For this review, use the dimensioned drawing (mm, ordinates from the lowest corner) and the shaded views. Give positions to 0.01 mm unless a question says otherwise; leave off trailing zeros. Write each loop counter-clockwise with the first axis right and the second up, starting at its lowest first coordinate (ties: lowest second). Pieces come first, ordered by that corner, then holes. Notation, with made-up numbers: (-6, 6) - (38, 6) arc R10 cw to (38, 18) - close; hole circle Ø5 at (25, 87). An arc over 180 degrees is marked (long way). One line per question, with ' | ' between items. Start each with the question number.
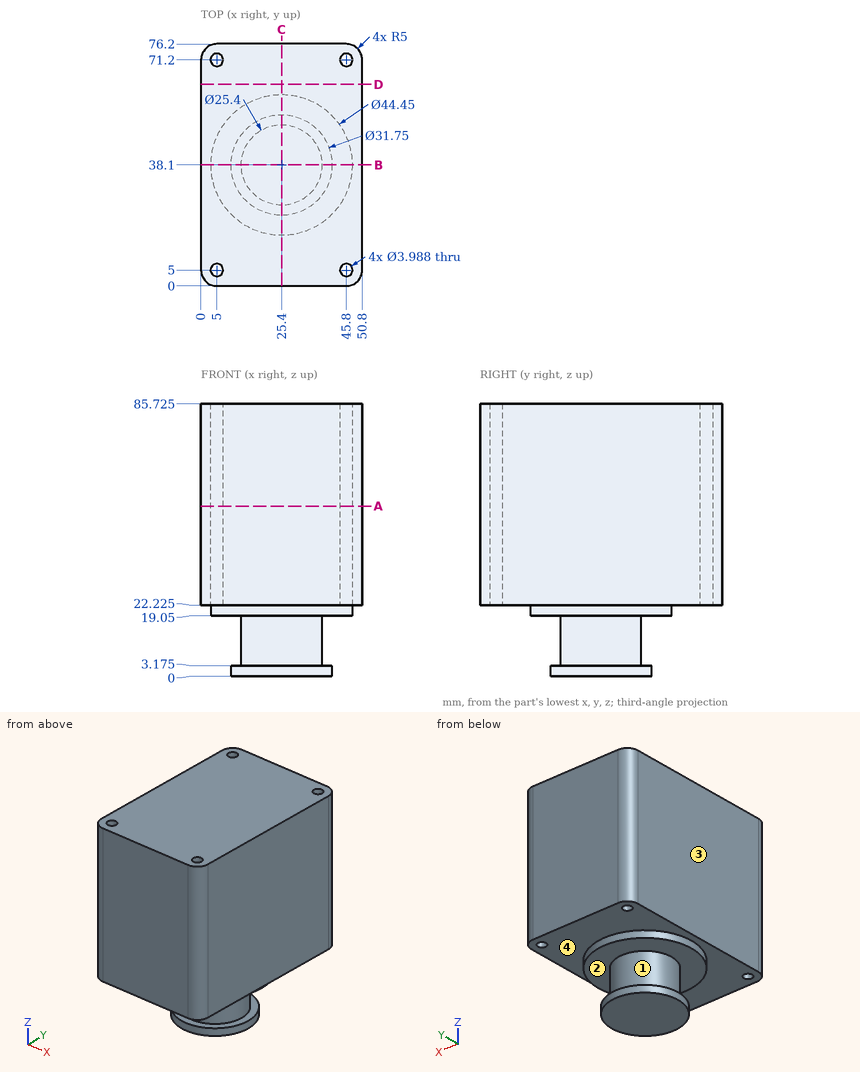
Item 1: Take a section at D-D (y = 63.5). Give the boundary of the cut face in (x, z) (3 decimals).
Item 2: The part is to be moulded in two halves that separate along Z. For the marked faces 1, 2, 3 and 4, say which applies: +Z half, -Z half, draft (parallel to the pull), parting line (faces both ways), or undercut.
Item 3: For probe 1 along Z at (x, y) = (36, 30) (3 decimals); probe 2 along Y at (x, z) = (6.5, 69); probe 3 along Z at (x, y) = (27.5, 64) (3 decimals), list the stretches that pass through material, from the lowest coordinate up.
Item 4: Take a section at B-B (y = 38.1). Give the boundary of the cut face in (x, z) (3 decimals), plus the area to 3 significant figures.
Item 5: Take a section at C-C (x = 25.4). Give the boundary of the cut face in (y, z) (3 decimals), plus the area to 3 significant figures.
Item 6: Clearance check with flat-ended pins moving along their axes: P1, Ø3.5, axis at x = 45.8, y = 71.2, coming from the +Z side; P2, Ø1, axis at x = 7, y = 43.5, coming from the -Z side. State where each tip first meets the part, or that it passes through.
Item 7: Take a section at A-A (z = 53.5). Give the boundary of the cut face in (x, y).
Check sheet entries:
1) outline: (0, 22.225) - (50.8, 22.225) - (50.8, 85.725) - (0, 85.725) - close
2) face 1: undercut | face 2: undercut | face 3: draft | face 4: -Z half
3) probe 1: z = 0 to 3.175, 19.05 to 85.725 | probe 2: y = 0 to 3.69, 6.31 to 69.89, 72.51 to 76.2 | probe 3: z = 22.225 to 85.725
4) outline: (0, 22.225) - (3.175, 22.225) - (3.175, 19.05) - (12.7, 19.05) - (12.7, 3.175) - (9.525, 3.175) - (9.525, 0) - (41.275, 0) - (41.275, 3.175) - (38.1, 3.175) - (38.1, 19.05) - (47.625, 19.05) - (47.625, 22.225) - (50.8, 22.225) - (50.8, 85.725) - (0, 85.725) - close | area: 3,870 mm^2
5) outline: (0, 22.225) - (15.875, 22.225) - (15.875, 19.05) - (25.4, 19.05) - (25.4, 3.175) - (22.225, 3.175) - (22.225, 0) - (53.975, 0) - (53.975, 3.175) - (50.8, 3.175) - (50.8, 19.05) - (60.325, 19.05) - (60.325, 22.225) - (76.2, 22.225) - (76.2, 85.725) - (0, 85.725) - close | area: 5,480 mm^2
6) P1: passes through | P2: stops at z = 19.05
7) outline: (0, 5) arc R5 ccw to (5, 0) - (45.8, 0) arc R5 ccw to (50.8, 5) - (50.8, 71.2) arc R5 ccw to (45.8, 76.2) - (5, 76.2) arc R5 ccw to (0, 71.2) - close; hole circle Ø3.99 at (5, 5); hole circle Ø3.99 at (5, 71.2); hole circle Ø3.99 at (45.8, 5); hole circle Ø3.99 at (45.8, 71.2)
